Work out the finished part from the listing and answer in its coordinate system (mm). A direction names the side the tool comes from. Coordinates: 2 decimals unless noted, no trailing zeros. Write each loop counter-clockwise with the first axis right and the second up, starting at its lowest first coordinate (ties: lowest second). Pieces come first, ordered by that corner, then holes. Notation, with made-up numbers: (83, -15.75) - (93, -15.75) arc R32 cw to (93, 18.25) - close; hole circle Ø1 at (30, 12). An arc over 180 degrees is marked (long way). Use one line per item in the form item = value. Start each with the question number.
Item 1: A cutting plane is placed at C-C (z = 36.5). Write down the section's boundary in (x, y).
Item 2: A cutting plane is placed at B-B (y = -6). Write down the section's boundary in (x, z) (3 decimals), then the cut area to 3 significant figures.
Item 3: For faces 1 (the flat face through (0, 0, -25.4)), 2 (the flat face through (10, 9, 50.8)), determine the directions among +Z, -Z, +X, -X, +Y, -Y from which every point of the face is accessible in a straight line to the end or side of a thin tool.
Item 4: A cutting plane is placed at A-A (x = 0). Write down the section's boundary in (y, z) (1 decimal).
Item 5: A cutting plane is placed at D-D (y = -14.5). Write down the section's boundary in (x, z) (3 decimals), then the cut area to 3 significant figures.
Item 6: Given pin 1 (2 mm diameter, centred on x = -2, z = -10.5, fed in from -Y); pin 2 (10 mm diameter, centred on x = 10.5, z = 29.5, fed in from -Y); pin 3 (10 mm diameter, centred on x = -17.5, y = 13.5, fed in from -Z); pin 4 (3 mm diameter, centred on x = 14.5, z = -4, fed in from -Y), each flat-ended and moving along its own axis, determine where each tip first touches the part or whether it passes through.
Item 7: Consider probe 1 along Z at (x, y) = (-11, -12.5) (3 decimals); probe 2 along Y at (x, z) = (-0.5, 16); probe 3 along Y at (x, z) = (-2, 6). Determine where each line is inside the solid, lowest interval first.
from build123d import *

# Parameters (mm, degrees)
F0_R          = 12.7
F1_DEPTH      = 25.4
F1_DEPTH_BACK = 50.8
F3_DEPTH      = 15.875


# Not quite as in the source:
# - a feature names something its author has since deleted; it is built from what else it names


with BuildPart() as f1:
    # F0 (on Top) → F1 (new body, two sides)
    with BuildSketch(Plane.XY) as f1_sk:
        Circle(F0_R)
    extrude(amount=-F1_DEPTH)
    extrude(f1_sk.sketch, amount=F1_DEPTH_BACK)

    # F2 (on face) → F3 (join)
    with BuildSketch(Plane.XY.offset(50.8)):
        Polygon((11.9150661804, 20.6375), (-11.9150661804, 20.6375), (-23.8301323608, 0), (-11.9150661804, -20.6375), (11.9150661804, -20.6375), (23.8301323608, 0), align=None)
    extrude(amount=F3_DEPTH)


solid = f1.part
Answer:
q1.outline = circle Ø25.4 at (0, 0)
q2.outline = (-20.366, 50.8) - (-11.193, 50.8) - (-11.193, -25.4) - (11.193, -25.4) - (11.193, 50.8) - (20.366, 50.8) - (20.366, 66.675) - (-20.366, 66.675) - close
q2.area = 2,350 mm²
q3.face_1 = -Z, +X, -X, +Y, -Y
q3.face_2 = -Z
q4.outline = (-20.6, 50.8) - (-12.7, 50.8) - (-12.7, -25.4) - (12.7, -25.4) - (12.7, 50.8) - (20.6, 50.8) - (20.6, 66.7) - (-20.6, 66.7) - close
q5.outline = (-15.459, 50.8) - (15.459, 50.8) - (15.459, 66.675) - (-15.459, 66.675) - close
q5.area = 491 mm²
q6.pin_1 = -12.66
q6.pin_2 = -11.45
q6.pin_3 = 50.8
q6.pin_4 = through
q7.probe_1 = 50.8 to 66.675
q7.probe_2 = -12.69 to 12.69
q7.probe_3 = -12.54 to 12.54
